```python
from build123d import *

# Parameters (mm, degrees)
SKETCH1_W           = 45
SKETCH1_H           = 45
BOSS_EXTRUDE1_DEPTH = 10
SKETCH2_R           = 1.5
CUT_EXTRUDE1_DEPTH  = 10
SKETCH3_R           = 1.5
CUT_EXTRUDE2_DEPTH  = 10


with BuildPart() as part:
    # Sketch1 → Boss-Extrude1 (new body)
    with BuildSketch(Plane.XY):
        Rectangle(SKETCH1_W, SKETCH1_H)
    extrude(amount=BOSS_EXTRUDE1_DEPTH)

    # Sketch2 → Cut-Extrude1 (cut)
    with BuildSketch(Plane.XY.offset(10)):
        with Locations((-12.5, 12.5)):
            Circle(SKETCH2_R)
        with Locations((12.5, 12.5)):
            Circle(SKETCH2_R)
        with Locations((12.5, -12.5)):
            Circle(SKETCH2_R)
        with Locations((-12.5, -12.5)):
            Circle(SKETCH2_R)
    extrude(amount=-CUT_EXTRUDE1_DEPTH, mode=Mode.SUBTRACT)

    # Sketch3 → Cut-Extrude2 (cut)
    with BuildSketch(Plane.XY.offset(10)):
        with Locations((-5, 5)):
            Circle(SKETCH3_R)
        with Locations((5, 5)):
            Circle(SKETCH3_R)
        with Locations((5, -5)):
            Circle(SKETCH3_R)
        with Locations((-5, -5)):
            Circle(SKETCH3_R)
    extrude(amount=-CUT_EXTRUDE2_DEPTH, mode=Mode.SUBTRACT)


solid = part.part
```
Can you work these out from the model? Positions are in its coordinate system, mm. Coordinates: 2 decimals unless noted, no trailing zeros. Loops run counter-clockwise (first coordinate to the right, second up) from the corner with the lowest first, then second, coordinate; pieces in that order, holes last. Notation, with made-up numbers: M 82,-1.75 L 113,-1.75 A17 cw 113,23.25 Z; hole C 3,57 d3. An arc over 180 degrees is marked long. Put each result on its own line as item: value. Start each with the question number.
(1) I need wall thicknesses on probe 1 along Y at (x, z) = (12.5, 4.5); probe 2 along Y at (x, z) = (5, 0.75); probe 3 along X at (y, z) = (12, 9.25). Which ranges of each line are inside material? Lowest first, please.
(2) Imagine slicing it at A-A on x = -5. List the corners of the cut face in (y, z) for me, and give its area (3 significant figures).
(3) Imagine slicing it at C-C on y = -12.5. List the corners of the cut face in (x, z) for me, and give its area (3 significant figures).
(4) Imagine slicing it at B-B on z = 4.25. Give the number of separate pieces and of enclosed holes in the cut face, and give its area (3 significant figures).
(5) We'd pull the mould along X, two halves only. Please class faces 1 (the face through (11, -12.43, 5.07)), 2 (the face through (0, 0, 0)), 3 (the face through (-22.5, 0, 5)): +X half, -X half, draft (parallel to the pull), parting line (faces both ways), or undercut.
Worked answers:
1. probe 1: y = -22.5 to -14, -11 to 11, 14 to 22.5
1. probe 2: y = -22.5 to -6.5, -3.5 to 3.5, 6.5 to 22.5
1. probe 3: x = -22.5 to -13.91, -11.09 to 11.09, 13.91 to 22.5
2. outline: M -22.5,0 L -6.5,0 L -6.5,10 L -22.5,10 Z; M -3.5,0 L 3.5,0 L 3.5,10 L -3.5,10 Z; M 6.5,0 L 22.5,0 L 22.5,10 L 6.5,10 Z
2. area: 390 mm2
3. outline: M -22.5,0 L -14,0 L -14,10 L -22.5,10 Z; M -11,0 L 11,0 L 11,10 L -11,10 Z; M 14,0 L 22.5,0 L 22.5,10 L 14,10 Z
3. area: 390 mm2
4. separate pieces: 1
4. enclosed holes: 8
4. area: 1,970 mm2
5. face 1: undercut
5. face 2: draft
5. face 3: -X half
